Can you work these out from the drawing? Everything is in mm from the part's minimum corner. Give positions to 0.01 mm unless a question says otherwise; leave off trailing zeros. Write each loop counter-clockwise with the first axis right and the second up, starting at its lowest first coordinate (ties: lowest second). Pieces come first, ordered by that corner, then holes. Notation, with made-up numbers: (-21, -7) -> (23, -7) arc R19 ccw to (23, 10) -> close; hole circle Ø1 at (81.25, 26.5). An arc over 180 degrees is marked (long way). Return JSON: item names as keys, results as strings.
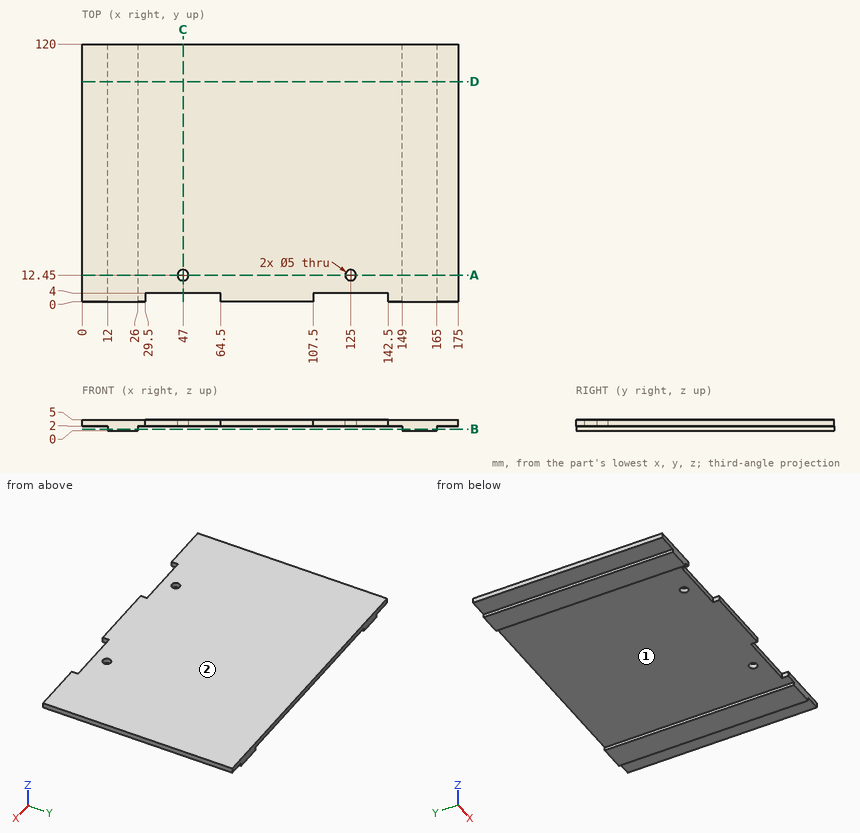
1. Suppose I cut it at C-C, the plane x = 47. List the corners of the cut face in (y, z) for me.
Taken from the geometry:
{"outline": "(4, 2) -> (9.95, 2) -> (9.95, 5) -> (4, 5) -> close; (14.95, 2) -> (120, 2) -> (120, 5) -> (14.95, 5) -> close"}
2. Suppose I cut it at A-A, the plane y = 12.45. List the corners of the cut face in (x, z) for me, and give its area (3 significant figures).
Taken from the geometry:
{"outline": "(0, 2) -> (12, 2) -> (12, 0) -> (26, 0) -> (26, 2) -> (44.5, 2) -> (44.5, 5) -> (0, 5) -> close; (49.5, 2) -> (122.5, 2) -> (122.5, 5) -> (49.5, 5) -> close; (127.5, 2) -> (149, 2) -> (149, 0) -> (165, 0) -> (165, 2) -> (175, 2) -> (175, 5) -> (127.5, 5) -> close", "area": "555 mm²"}
3. For pin 1 Ø0.6 at (y, z) = (78.5, 1.5) entering from -X; pin 2 Ø0.9 at (x, z) = (44.5, 4) entering from -Y; pin 3 Ø3 at (x, y) = (34.5, 98) entering from -Z, each with a flat end and sliding along its axis, tell me the tip position at first contact or that it passes through.
Taken from the geometry:
{"pin 1": "stops at x = 12", "pin 2": "stops at y = 4", "pin 3": "stops at z = 2"}
4. Suppose I cut it at D-D, the plane y = 102.5. List the corners of the cut face in (x, z) for me, and give its area (3 significant figures).
Taken from the geometry:
{"outline": "(0, 2) -> (12, 2) -> (12, 0) -> (26, 0) -> (26, 2) -> (149, 2) -> (149, 0) -> (165, 0) -> (165, 2) -> (175, 2) -> (175, 5) -> (0, 5) -> close", "area": "585 mm²"}
5. If we mould it in two halves opening along X, with no side actions, what happens to the marked faces 1 and 2? For each: released by +X, released by -X, zero draft, split by the parting line, or undercut.
Taken from the geometry:
{"face 1": "undercut", "face 2": "zero draft"}
6. Suppose I cut it at B-B, the plane z = 0.75. List the corners of the cut face in (x, y) for me.
Taken from the geometry:
{"outline": "(12, 0) -> (26, 0) -> (26, 120) -> (12, 120) -> close; (149, 0) -> (165, 0) -> (165, 120) -> (149, 120) -> close"}
7. If I drill on line 1 (Y direction, x = 47, z = 3.4); line 2 (Z direction, x = 85, y = 41); line 3 (Y direction, x = 132.5, z = 2.5), over which ranges is the centre line in solid material (lowest first)? Write a range as [from, to].
Taken from the geometry:
{"line 1": "y = [4, 9.95], [14.95, 120]", "line 2": "z = [2, 5]", "line 3": "y = [4, 120]"}
